The listing builds one solid part. Answer for the finished solid, in the listing's coordinates (mm). Face numbers are marked on the shaded views. A direction names the side the tool comes from. Round coordinates to 2 decimals unless told otherwise and drop trailing zeros. Loops run counter-clockwise (first coordinate to the right, second up) from the corner with the lowest first, then second, coordinate; pieces in that order, holes last. Notation, with made-up numbers: (31, 5) -> (51, 5) arc R26 cw to (51, 24) -> close; hole circle Ø1 at (10.25, 19). An arc over 180 degrees is marked (long way). Use a Markdown table: item, result. Add a question column.
Q1. For a pull along X with two mould halves and no side action, classify the marked faces 4, 5, 6 and 7 as released by +X, released by -X, zero draft, split by the parting line, or undercut.
Q2. Section B-B on y = -30.5 is taken. Give the vertices of the cut face in (x, z), then the cut area to 3 significant figures.
Q3. Given pin 1 Ø2.5 at (x, y) = (20, -30.5) entering from -Z; pin 2 Ø1.5 at (x, y) = (12.5, -43) entering from +Z; pin 3 Ø4 at (x, y) = (18, -41.5) entering from +Z; pin 4 Ø4.5 at (x, y) = (20, -30.5) entering from -Z, each flat-ended and moving along its own axis, determine where each tip first touches the part or whether it passes through.
Q4. Section A-A on z = 15 is taken. Give the vertices of the cut face in (x, y), then the cut area to 3 significant figures.
Q5. Section D-D on y = -41.5 is taken. Give the vertices of the cut face in (x, z).
Q6. Consider line 1 (X direction, y = -30.5, z = 1.1); line 2 (Y direction, x = 8, z = 21.75); line 3 (Y direction, x = 5, z = 2.7). Determine where each line is inside the solid, lowest interval first.
Q7. Which of the six approach directions +Z, -Z, +X, -X, +Y, -Y give full straight-line access (tool end or side, diameter ignored) to the marked faces 1, 2 and 3?
Q8. Section C-C on x = 5 is taken. Give the vertices of the cut face in (y, z), then the cut area to 3 significant figures.
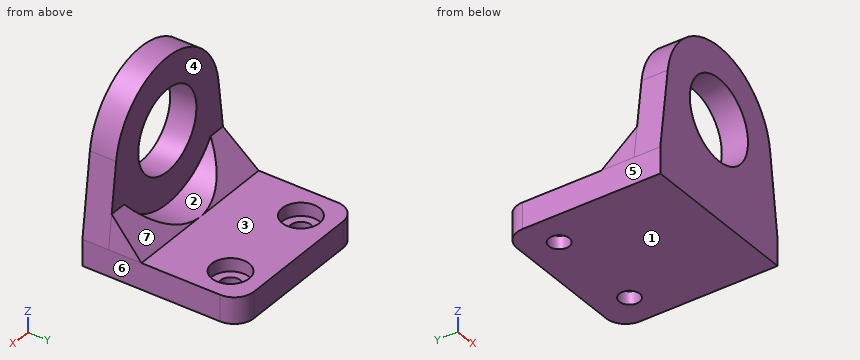
from build123d import *

# Parameters (mm, degrees)
SKETCH1_W           = 25
SKETCH1_H           = 10
SKETCH1_R           = 1.55
BOSS_EXTRUDE1_DEPTH = 4
SKETCH2_W           = 25
SKETCH2_H           = 4
BOSS_EXTRUDE2_DEPTH = 10
SKETCH3_R           = 6.2
BOSS_EXTRUDE3_DEPTH = 4
CHAMFER1_SIZE       = 5
CUT_EXTRUDE1_START  = 10
SKETCH4_R           = 11
CUT_EXTRUDE1_DEPTH  = 10
FILLET1_R           = 3
SKETCH5_R           = 2.85
CUT_EXTRUDE2_DEPTH  = 2


with BuildPart() as part:
    # Sketch1 → Boss-Extrude1 (new body)
    with BuildSketch(Plane.XY):
        with Locations((12.5, -30.5)):
            Rectangle(SKETCH1_W, SKETCH1_H)
        with Locations((5, -30.5)):
            Circle(SKETCH1_R, mode=Mode.SUBTRACT)
        with Locations((20, -30.5)):
            Circle(SKETCH1_R, mode=Mode.SUBTRACT)
    extrude(amount=BOSS_EXTRUDE1_DEPTH)

    # Sketch2 → Boss-Extrude2 (add)
    with BuildSketch(Plane.XZ.offset(35.5)):
        with Locations((12.5, 2)):
            Rectangle(SKETCH2_W, SKETCH2_H)
    extrude(amount=BOSS_EXTRUDE2_DEPTH)

    # Sketch3 → Boss-Extrude3 (add)
    with BuildSketch(Plane.XZ.offset(45.5)):
        with BuildLine():
            Line((0, 4), (1.589269612, 16.398557259))
            ThreePointArc((1.589269612, 16.398557259), (12.5, 26), (23.410730388, 16.398557259))
            Line((23.410730388, 16.398557259), (25, 4))
            Line((25, 4), (25, 0))
            Line((25, 0), (0, 0))
            Line((0, 0), (0, 4))
        make_face()
        with Locations(Location((12.5, 15, 0), (0, 0, 270))):
            Circle(SKETCH3_R, mode=Mode.SUBTRACT)
    extrude(amount=BOSS_EXTRUDE3_DEPTH)

    # Chamfer1
    # the kernel refuses this chamfer: 5 mm, written as the material it adds along each edge
    with BuildSketch(Plane(origin=(25, -45.5, 4), x_dir=(0, 0.9996219169112968, -0.027495876610586403), z_dir=(-1, 0, 0))) as chamfer1_piece_1_section:
        Polygon((CHAMFER1_SIZE * 0.999621916911, -CHAMFER1_SIZE * 0.0274958766106), (-CHAMFER1_SIZE * 0.0274958766106, -CHAMFER1_SIZE * 0.999621916911), (0, 0), align=None)
    chamfer1_piece_1 = extrude(amount=25, mode=Mode.PRIVATE)
    chamfer1_piece_1 = split(chamfer1_piece_1, bisect_by=Plane(origin=(24.592329288, -43.84115056, 7.18040981), z_dir=(-0.9918845807033364, 0, -0.12714156898106382)), keep=Keep.TOP, mode=Mode.PRIVATE)
    chamfer1_piece_1 = split(chamfer1_piece_1, bisect_by=Plane(origin=(0.407670712, -43.84115056, 7.18040981), z_dir=(0.9918845807033364, 0, -0.12714156898106413)), keep=Keep.TOP, mode=Mode.PRIVATE)
    chamfer1_piece_1 = chamfer1_piece_1 - Plane(origin=(12.5, -43.84115056, 15), x_dir=(0, 0, -1), z_dir=(0, 1, 0)) * Cylinder(6.2, 70, mode=Mode.PRIVATE)
    add(chamfer1_piece_1)

    # Sketch4 → Cut-Extrude1 (cut)
    with BuildSketch(Plane(origin=(0, -45.5, 0), x_dir=(1, 0, 0), z_dir=(0, 1, 0)).offset(CUT_EXTRUDE1_START)):
        with Locations((12.5, -15)):
            Circle(SKETCH4_R)
    extrude(amount=-CUT_EXTRUDE1_DEPTH, mode=Mode.SUBTRACT)

    # Fillet1
    fillet1_edges = [part.edges().sort_by_distance(p)[0] for p in [
        (25, -25.5, 2),
        (0, -25.5, 2),
    ]]
    fillet(fillet1_edges, radius=FILLET1_R)

    # Sketch5 → Cut-Extrude2 (cut)
    with BuildSketch(Plane.XY.offset(4)):
        with Locations((20, -30.5)):
            Circle(SKETCH5_R)
        with Locations((5, -30.5)):
            Circle(SKETCH5_R)
    extrude(amount=-CUT_EXTRUDE2_DEPTH, mode=Mode.SUBTRACT)


solid = part.part
Checked values:
| question | item | result |
|---|---|---|
| 1 | face 4 | undercut |
| 1 | face 5 | released by -X |
| 1 | face 6 | released by +X |
| 1 | face 7 | zero draft |
| 2 | outline | (0, 0) -> (3.45, 0) -> (3.45, 2) -> (2.15, 2) -> (2.15, 4) -> (0, 4) -> close; (6.55, 0) -> (18.45, 0) -> (18.45, 2) -> (17.15, 2) -> (17.15, 4) -> (7.85, 4) -> (7.85, 2) -> (6.55, 2) -> close; (21.55, 0) -> (25, 0) -> (25, 4) -> (22.85, 4) -> (22.85, 2) -> (21.55, 2) -> close |
| 2 | area | 64.8 mm2 |
| 3 | pin 1 | passes through |
| 3 | pin 2 | stops at z = 4.03 |
| 3 | pin 3 | stops at z = 6.43 |
| 3 | pin 4 | stops at z = 0 |
| 4 | outline | (1.41, -49.5) -> (6.3, -49.5) -> (6.3, -45.5) -> (1.41, -45.5) -> close; (18.7, -49.5) -> (23.59, -49.5) -> (23.59, -45.5) -> (18.7, -45.5) -> close |
| 4 | area | 39.1 mm2 |
| 5 | outline | (0, 0) -> (25, 0) -> (25, 4) -> (24.87, 5) -> (17.08, 5) arc R11 cw to (7.92, 5) -> (0.13, 5) -> (0, 4) -> close |
| 6 | line 1 | x = 0 to 3.45, 6.55 to 18.45, 21.55 to 25 |
| 6 | line 2 | y = -49.5 to -45.5 |
| 6 | line 3 | y = -49.5 to -33.35, -27.65 to -25.5 |
| 7 | face 1 | -Z, +X, -X, +Y, -Y |
| 7 | face 2 | +Z, +Y |
| 7 | face 3 | +Z, +X, -X, +Y |
| 8 | outline | (-49.5, 0) -> (-32.05, 0) -> (-32.05, 2) -> (-33.35, 2) -> (-33.35, 4) -> (-40.5, 4) -> (-43.45, 6.95) -> (-45.5, 6.95) -> (-45.5, 23.05) -> (-49.5, 23.05) -> close; (-28.95, 0) -> (-25.5, 0) -> (-25.5, 4) -> (-27.65, 4) -> (-27.65, 2) -> (-28.95, 2) -> close |
| 8 | area | 165 mm2 |
